Geometry check sheet. Reference: the model listing, model coordinates, mm. Face numbers are marked on the shaded views. A direction names the side the tool comes from. Give positions to 0.01 mm unless a question says otherwise; leave off trailing zeros. Order: outer loops, then holes, each group sorted by start corner. A loop starts at its lowest first (then second) coordinate and runs counter-clockwise, first axis right, second up.
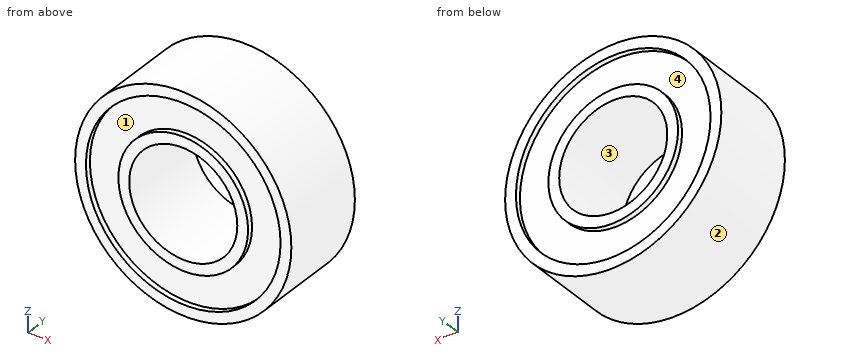
from build123d import *

# Parameters (mm, degrees)
SKETCH1_R           = 5
SKETCH1_R_2         = 2.5
BOSS_EXTRUDE1_DEPTH = 2
SKETCH2_R           = 4.5
SKETCH2_R_2         = 3
CUT_EXTRUDE1_DEPTH  = 0.25


with BuildPart() as part:
    # Sketch1 → Boss-Extrude1 (new body, symmetric)
    with BuildSketch(Plane(origin=(0, 0, 0), x_dir=(1, 0, 0), z_dir=(0, 1, 0))):
        Circle(SKETCH1_R)
        Circle(SKETCH1_R_2, mode=Mode.SUBTRACT)
    extrude(amount=BOSS_EXTRUDE1_DEPTH, both=True)

    # Sketch2 → Cut-Extrude1 (cut)
    with BuildSketch(Plane(origin=(0, 2, 0), x_dir=(1, 0, 0), z_dir=(0, 1, 0))):
        Circle(SKETCH2_R)
        Circle(SKETCH2_R_2, mode=Mode.SUBTRACT)
    cut_extrude1 = extrude(amount=-CUT_EXTRUDE1_DEPTH, mode=Mode.SUBTRACT)

    # Mirror1: Cut-Extrude1 across plane
    add(cut_extrude1.mirror(Plane.ZX), mode=Mode.SUBTRACT)


solid = part.part
Item 1: Gauge pin test, flat ends, axial feed: pin 1 (2 mm diameter, centred on x = 0.5, z = 0, fed in from -Y) (3 decimals); pin 2 (2 mm diameter, centred on x = 2, y = -1, fed in from +Z). Record the tip position at first contact, or that the pin passes through.
Reported:
pin 1: passes through
pin 2: stops at z = 4.9
Item 2: Set-up check for the marked faces 3 and 4: record each of +Z, -Z, +X, -X, +Y, -Y from which the full face is reachable in a straight line by a thin tool's end or side.
Reported:
face 3: +Y, -Y
face 4: +Y
Item 3: Sectioned sample at D-D (y = 0.25). Enter the section's corners in (x, z).
Reported:
outline: circle Ø10 at (0, 0); hole circle Ø5 at (0, 0)
Item 4: Scan lines: L1, parallel to Z at x = 0, y = -1.9; L2, parallel to Z at x = 0, y = 0. Record each from-to range of solid material in increasing order.
Reported:
L1: z = -5 to -4.5, -3 to -2.5, 2.5 to 3, 4.5 to 5
L2: z = -5 to -2.5, 2.5 to 5
Item 5: Sectioned sample at A-A (x = 0). Enter the section's corners in (y, z), and give its area (3 significant figures).
Reported:
outline: (-2, -5) - (2, -5) - (2, -4.5) - (1.75, -4.5) - (1.75, -3) - (2, -3) - (2, -2.5) - (-2, -2.5) - (-2, -3) - (-1.75, -3) - (-1.75, -4.5) - (-2, -4.5) - close; (-2, 2.5) - (2, 2.5) - (2, 3) - (1.75, 3) - (1.75, 4.5) - (2, 4.5) - (2, 5) - (-2, 5) - (-2, 4.5) - (-1.75, 4.5) - (-1.75, 3) - (-2, 3) - close
area: 18.5 mm2
Item 6: Sectioned sample at C-C (x = -3.25). Enter the section's corners in (y, z).
Reported:
outline: (-2, -3.8) - (2, -3.8) - (2, -3.11) - (1.75, -3.11) - (1.75, 3.11) - (2, 3.11) - (2, 3.8) - (-2, 3.8) - (-2, 3.11) - (-1.75, 3.11) - (-1.75, -3.11) - (-2, -3.11) - close
Item 7: Sectioned sample at B-B (z = 0). Enter the section's corners in (x, y), and give its area (3 significant figures).
Reported:
outline: (-5, -2) - (-4.5, -2) - (-4.5, -1.75) - (-3, -1.75) - (-3, -2) - (-2.5, -2) - (-2.5, 2) - (-3, 2) - (-3, 1.75) - (-4.5, 1.75) - (-4.5, 2) - (-5, 2) - close; (2.5, -2) - (3, -2) - (3, -1.75) - (4.5, -1.75) - (4.5, -2) - (5, -2) - (5, 2) - (4.5, 2) - (4.5, 1.75) - (3, 1.75) - (3, 2) - (2.5, 2) - close
area: 18.5 mm2
Item 8: Draft check along X on the marked faces 1 and 2. Enter one of: released by +X, released by -X, zero draft, split by the parting line, or undercut.
Reported:
face 1: undercut
face 2: split by the parting line
